The drawing under review shows one solid part. Ordinate dimensions are in mm from its lowest x, y, z. A direction names the side the tool comes from. Give positions to 0.01 mm unless a question says otherwise; leave off trailing zeros. Order: outer loops, then holes, each group sorted by start corner. A loop starts at its lowest first (then second) coordinate and runs counter-clockwise, first axis right, second up. Notation, with made-up numbers: (31.5, 61.25) - (58.5, 61.25) arc R20 cw to (58.5, 90.25) - close; hole circle Ø11 at (45, 25). An arc over 180 degrees is marked (long way). Write item = value, one per line. Start each with the question number.
1. For P1, Ø24.5, axis at x = 22, y = 24.5, coming from the +Z side; P2, Ø3, axis at y = 12.5, z = 9.5, coming from the +X side; P3, Ø8, axis at x = 33.5, z = 11.5, coming from the +Y side; P4, Ø3, axis at x = 21.5, z = 10.5, coming from the -Y side, all flat-tipped, find the tip position at first contact; note any pin that passes through.
2. Wall thickness on probe 1 along Y at (x, z) = (13, 14.5); probe 2 along Z at (x, y) = (23, 33.5); probe 3 along Y at (x, z) = (42.5, 5.25): over which ranges is each line inside the solid? List them lowest first.
3. We need section A-A, the plane x = 25. Give the boundary of the cut face in (y, z).
4. We need section B-B, the plane y = 25. Give the boundary of the cut face in (x, z).
5. We need section C-C, the plane x = 30. Give the boundary of the cut face in (y, z), and give its area (3 significant figures).
6. Machinability: for the marked faces 1 and 2, which of the approach directions +Z, -Z, +X, -X, +Y, -Y give a long, thin tool a straight path to every point of the face, cutting with its end or side? Answer none if there is none.
7. Mouldability with a two-part tool opening along Y and no side actions: class the marked faces 3, 4, 5 and 6 as pulls with the +Y half, pulls with the -Y half, needs draft (parallel to the pull), parting line crosses it, or undercut.
8. We need section D-D, the plane y = 8. Give the boundary of the cut face in (x, z), and give its area (3 significant figures).
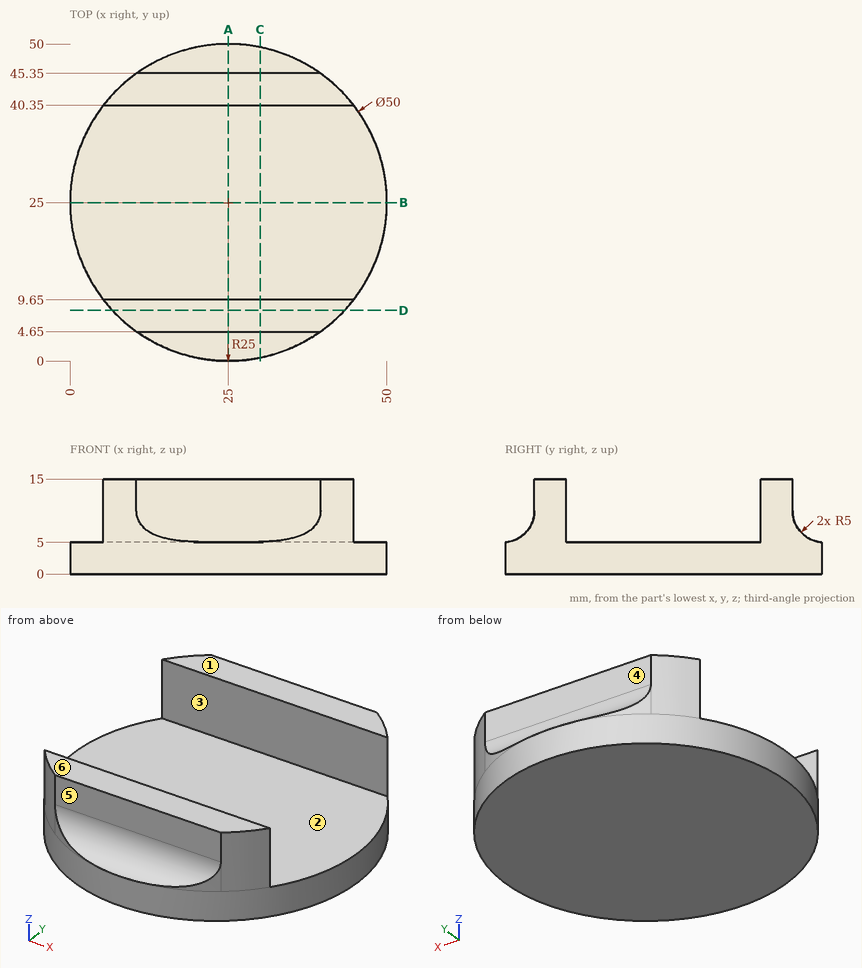
Model answer:
q1.P1 = 5
q1.P2 = through
q1.P3 = 46.02
q1.P4 = 4.55
q2.probe_1 = 4.65 to 9.65, 40.35 to 45.35
q2.probe_2 = 0 to 5
q2.probe_3 = 7.15 to 9.65, 40.35 to 42.85
q3.outline = (0, 0) - (50, 0) - (50, 5.01) arc R5 cw to (45.35, 10) - (45.35, 15) - (40.35, 15) - (40.35, 5) - (9.65, 5) - (9.65, 15) - (4.65, 15) - (4.65, 10) arc R5 cw to (0, 5.01) - close
q4.outline = (0, 0) - (50, 0) - (50, 5) - (0, 5) - close
q5.outline = (0.51, 0) - (49.49, 0) - (49.49, 5.07) arc R5 cw to (45.35, 10) - (45.35, 15) - (40.35, 15) - (40.35, 5) - (9.65, 5) - (9.65, 15) - (4.65, 15) - (4.65, 10) arc R5 cw to (0.51, 5.07) - close
q5.area = 356 mm2
q6.face_1 = +Z, +X, -X, +Y, -Y
q6.face_2 = +Z, +X, -X
q7.face_3 = undercut
q7.face_4 = pulls with the +Y half
q7.face_5 = pulls with the -Y half
q7.face_6 = needs draft
q8.outline = (6.67, 0) - (43.33, 0) - (43.33, 15) - (6.67, 15) - close
q8.area = 550 mm2
